Verification items for the finished model (mm, model axes). A direction names the side the tool comes from. Give positions to 0.01 mm unless a question says otherwise; leave off trailing zeros. Loops run counter-clockwise (first coordinate to the right, second up) from the corner with the lowest first, then second, coordinate; pieces in that order, holes last. Notation, with made-up numbers: (-36.5, -7) - (-26.5, -7) arc R23 cw to (-26.5, 12) - close; hole circle Ø11 at (62, -6). An arc over 180 degrees is marked (long way). Use one line per item in the form item = value.
```python
from build123d import *

# Parameters (mm, degrees)
SKETCH_1_W      = 4.3
SKETCH_1_H      = 8
EXTRUDE_1_DEPTH = 5
EXTRUDE_2_DEPTH = 4.3
SKETCH_3_R      = 1
EXTRUDE_3_DEPTH = 4.3


with BuildPart() as part:
    # 草图1 → 凸台-拉伸1 (new body)
    with BuildSketch(Plane(origin=(0, 0, 0), x_dir=(1, 0, 0), z_dir=(0, 1, 0))):
        Rectangle(SKETCH_1_W, SKETCH_1_H)
    extrude(amount=EXTRUDE_1_DEPTH)

    # 草图2 → 凸台-拉伸2 (add)
    with BuildSketch(Plane(origin=(2.15, 0, 0), x_dir=(0, 0, -1), z_dir=(1, 0, 0))):
        with BuildLine():
            Line((-4, 2), (-7, 2))
            add(Edge.make_bspline(
                [(-7, 2), (-6.002659385, 0.317190086), (-4, 0)],
                knots=[0, 0, 0, 1, 1, 1], degree=2))
            Line((-4, 0), (-4, 2))
        make_face()
        with BuildLine():
            Line((4, 2), (7, 2))
            add(Edge.make_bspline(
                [(4, 0), (5.86881421, 0.295991093), (7, 2)],
                knots=[0, 0, 0, 1, 1, 1], degree=2))
            Line((4, 0), (4, 2))
        make_face()
    extrude(amount=-EXTRUDE_2_DEPTH)

    # 草图3 → 凸台-拉伸3 (add)
    with BuildSketch(Plane(origin=(2.15, 0, 0), x_dir=(0, 0, -1), z_dir=(1, 0, 0))):
        with BuildLine():
            Line((-4, 5), (-0.782236668, 8.747328908))
            ThreePointArc((-0.782236668, 8.747328908), (1.909340646, 9.896542185), (4.322038795, 8.239989368))
            Line((4.322038795, 8.239989368), (4.184905625, 7.825161592))
            Line((4.184905625, 7.825161592), (4.528840035, 7.711464249))
            Line((4.528840035, 7.711464249), (4.35687283, 7.38145986))
            Line((4.35687283, 7.38145986), (4.638246106, 7.099532702))
            Line((4.638246106, 7.099532702), (4.35687283, 6.81871222))
            Line((4.35687283, 6.81871222), (4.628943103, 6.546106378))
            Line((4.628943103, 6.546106378), (4.35687283, 6.274570623))
            Line((4.35687283, 6.274570623), (4.492907966, 5.919485397))
            Line((4.492907966, 5.919485397), (4.184905625, 5.801487977))
            Line((4.184905625, 5.801487977), (4.3080813, 5.479969112))
            Line((4.3080813, 5.479969112), (4, 5))
            Line((4, 5), (-4, 5))
        make_face()
        with Locations((1.608881666, 6.873664454)):
            Circle(SKETCH_3_R, mode=Mode.SUBTRACT)
    extrude(amount=-EXTRUDE_3_DEPTH)


solid = part.part
```
1. Draft check along Y on faces 1 (the cylindrical face through (0.03, 5.897, -1.392)), 2 (the flat face through (0, 3, 4)), 3 (the flat face through (0, 0, 0)). Enter one of: released by +Y, released by -Y, zero draft, split by the parting line, or undercut.
Result set:
face_1 = undercut
face_2 = zero draft
face_3 = released by -Y
2. Depth check by flat-ended pin: pin 1 Ø1.5 at (x, z) = (1, -6) entering from +Y; pin 2 Ø0.9 at (x, y) = (0, 3.5) entering from -Z; pin 3 Ø2.5 at (x, y) = (-0.5, 4) entering from +Z. Enter the tip coordinate at first touch or a pass-through.
Result set:
pin_1 = 2
pin_2 = -4
pin_3 = 4
3. Section check C-C, the plane z = 3.25. Record the cut outline in (x, y).
Result set:
outline = (-2.15, 0) - (2.15, 0) - (2.15, 5.87) - (-2.15, 5.87) - close
4. Tool access check on faces 4 (the flat face through (0, 2, 5)), 5 (the flat face through (0, 2, -5)), 6 (the flat face through (-2.15, 4, 0)). Record the directions out of +Z, -Z, +X, -X, +Y, -Y that give a thin tool (end or side, any length) a straight path to the whole face; none if there is none.
Result set:
face_4 = +Z, +X, -X, +Y
face_5 = -Z, +X, -X
face_6 = +Z, -Z, -X, +Y, -Y
5. Section check B-B, the plane y = 4.75. Record the cut outline in (x, z).
Result set:
outline = (-2.15, -4) - (2.15, -4) - (2.15, 4) - (-2.15, 4) - close
6. Scan lines: probe 1 along Z at (x, y) = (0.65, 6.5); probe 2 along Z at (x, y) = (-0.45, 4); probe 3 along Y at (x, z) = (0.55, 3.25). Record each from-to range of solid material in increasing order.
Result set:
probe_1 = -4.58 to -2.54, -0.68 to 2.71
probe_2 = -4 to 4
probe_3 = 0 to 5.87
7. Section check A-A, the plane z = -1.5. Record the cut outline in (x, y), then the cut area to 3 significant figures.
Result set:
outline = (-2.15, 0) - (2.15, 0) - (2.15, 5.88) - (-2.15, 5.88) - close; (-2.15, 7.87) - (2.15, 7.87) - (2.15, 9.91) - (-2.15, 9.91) - close
area = 34.1 mm²
